Model file for the job. Use its own axes, mm. Coordinates: 2 decimals unless noted, no trailing zeros. Order: outer loops, then holes, each group sorted by start corner. A loop starts at its lowest first (then second) coordinate and runs counter-clockwise, first axis right, second up. Notation, with made-up numbers: (59, 13) -> (79, 13) arc R17 cw to (79, 34) -> close; hole circle Ø4 at (-19, -19). An arc over 180 degrees is marked (long way). Write item = value, one per line. Start each with the question number.
Q1. Wall check: line 1 (Y direction, x = 270.7, z = 3.25); line 2 (Y direction, x = -114, z = 3); line 3 (Y direction, x = -23, z = 2.75). Give the ranges that are in metal, low to high. Write a range as from..to.
Q2. Flat gauge pins, fed straight in: pin 1 (3 mm diameter, centred on y = -31, z = 2, fed in from +X); pin 2 (5.5 mm diameter, centred on x = 45.6, y = -19.2, fed in from -Z); pin 3 (2 mm diameter, centred on x = -57, z = 5, fed in from -Y); pin 4 (1 mm diameter, centred on y = -0.5, z = 2, fed in from -X). Where does each tip first touch, or does it go through?
Q3. Cut at B-B, the plane x = 89. List the corners of the cut face in (y, z), plus the area to 3 significant figures.
Q4. Cut at A-A, the plane z = 4.25. List the corners of the cut face in (x, y).
from build123d import *

# Parameters (mm, degrees)
SKETCH1_R           = 2.5
SKETCH1_R_2         = 3
BOSS_EXTRUDE1_DEPTH = 6.2


with BuildPart() as part:
    # Sketch1 → Boss-Extrude1 (new body)
    with BuildSketch(Plane.XY):
        with BuildLine():
            Line((85.6, -33.2), (-2.718519223, -20.878508118))
            ThreePointArc((-2.718519223, -20.878508118), (-8.41017463, -20.715920511), (-14, -21.8))
            Line((-14, -21.8), (-42.039824529, -38.092696265))
            ThreePointArc((-42.039824529, -38.092696265), (-46.884666341, -40.111316958), (-52.087842039, -40.8))
            Line((-52.087842039, -40.8), (-81.699109919, -40.8))
            ThreePointArc((-81.699109919, -40.8), (-91.370795398, -43.36753119), (-98.495572761, -50.394))
            ThreePointArc((-98.495572761, -50.394), (-129.24406218, -50.82175889), (-115.5, -23.312608885))
            Line((-115.5, -23.312608885), (-95.618089435, -21.65))
            ThreePointArc((-95.618089435, -21.65), (-78.309182519, -16.601252711), (-64.341378668, -5.2))
            ThreePointArc((-64.341378668, -5.2), (-61.413749232, -2.21456762), (-58, 0.2))
            ThreePointArc((-58, 0.2), (-29.282001226, 11.518177334), (1.5, 13.818827736))
            ThreePointArc((1.5, 13.818827736), (139.454874424, 0.958251967), (274.87829908, -28.323787594))
            ThreePointArc((274.87829908, -28.323787594), (283.738974288, -51.630641354), (258.857280718, -53.25))
            ThreePointArc((258.857280718, -53.25), (172.558903288, -40.371111866), (85.6, -33.2))
        make_face()
        with Locations(Location((-114, -41.25, 0), (0, 0, 180))):
            Circle(SKETCH1_R, mode=Mode.SUBTRACT)
        with Locations(Location((-47, -18.8, 0), (0, 0, 180))):
            Circle(SKETCH1_R_2, mode=Mode.SUBTRACT)
        with Locations(Location((45.6, -19.2, 0), (0, 0, 180))):
            Circle(SKETCH1_R_2, mode=Mode.SUBTRACT)
        with Locations(Location((0, 0, 0), (0, 0, 180))):
            Circle(SKETCH1_R_2, mode=Mode.SUBTRACT)
        with Locations(Location((270.7, -43.25, 0), (0, 0, 180))):
            Circle(SKETCH1_R_2, mode=Mode.SUBTRACT)
        with BuildLine():
            ThreePointArc((226.744224082, -27.259797753), (211.929816899, -23.860779344), (197.071572094, -20.658819377))
            ThreePointArc((197.071572094, -20.658819377), (190.434794526, -25.546132018), (195.40651845, -32.119913468))
            ThreePointArc((195.40651845, -32.119913468), (210.197393834, -34.160215491), (224.964543777, -36.365688118))
            ThreePointArc((224.964543777, -36.365688118), (230.232403999, -32.668395241), (226.744224082, -27.259797753))
        make_face(mode=Mode.SUBTRACT)
        with BuildLine():
            ThreePointArc((132.347185699, -9.089339403), (122.571709195, -15.840894216), (130.010518711, -25.104130489))
            ThreePointArc((130.010518711, -25.104130489), (147.296090717, -26.642266435), (164.560225388, -28.404797523))
            ThreePointArc((164.560225388, -28.404797523), (172.152990765, -22.51669502), (166.534944909, -14.721991823))
            ThreePointArc((166.534944909, -14.721991823), (149.462384392, -11.776267989), (132.347185699, -9.089339403))
        make_face(mode=Mode.SUBTRACT)
    extrude(amount=BOSS_EXTRUDE1_DEPTH)


solid = part.part
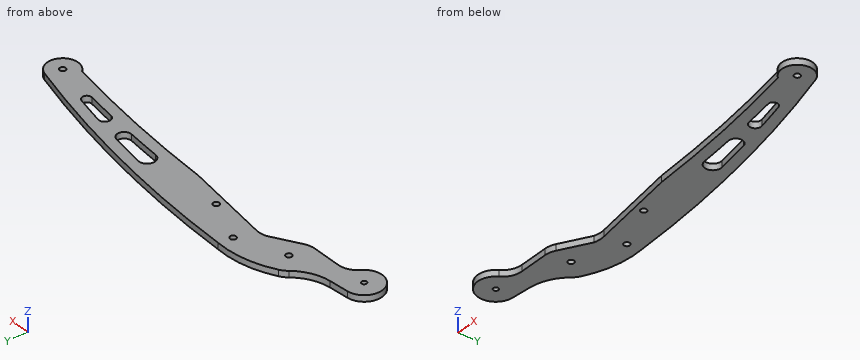
Here are the results:
q1.line_1 = -58.75..-46.25, -40.25..-27.16
q1.line_2 = -59.25..-43.75, -38.75..-23.19
q1.line_3 = -27.03..12.75
q2.pin_1 = 281.87
q2.pin_2 = through
q2.pin_3 = -40.8
q2.pin_4 = -59.86
q3.outline = (-33.37, 0) -> (7.6, 0) -> (7.6, 6.2) -> (-33.37, 6.2) -> close
q3.area = 254 mm²
q4.outline = (-115.5, -23.31) arc R18 ccw (long way) to (-98.5, -50.39) arc R19.5 cw to (-81.7, -40.8) -> (-52.09, -40.8) arc R20 ccw to (-42.04, -38.09) -> (-14, -21.8) arc R25.92 cw to (-2.72, -20.88) -> (85.6, -33.2) arc R1325 cw to (258.86, -53.25) arc R15.5 ccw (long way) to (274.88, -28.32) arc R1155.37 ccw to (1.5, 13.82) arc R103 ccw to (-58, 0.2) arc R23.32 ccw to (-64.34, -5.2) arc R45.29 cw to (-95.62, -21.65) -> close; hole circle Ø5 at (-114, -41.25); hole circle Ø6 at (-47, -18.8); hole circle Ø6 at (0, 0); hole circle Ø6 at (45.6, -19.2); hole (130.01, -25.1) arc R1336 cw to (164.56, -28.4) arc R6.92 ccw to (166.53, -14.72) arc R1144.37 ccw to (132.35, -9.09) arc R8.11 ccw (long way) to start; hole (195.41, -32.12) arc R1336 cw to (224.96, -36.37) arc R4.64 ccw to (226.74, -27.26) arc R1144.37 ccw to (197.07, -20.66) arc R5.79 ccw (long way) to start; hole circle Ø6 at (270.7, -43.25)
